Input: part model. Units: mm. Frame: model coordinates. A direction names the side the tool comes from. Coordinates: 2 decimals unless noted, no trailing zeros. Order: outer loops, then holes, each group sorted by start corner. A loop starts at its lowest first (then second) coordinate and runs counter-clockwise, first axis right, second up. Notation, with made-up numbers: (55, 51) -> (67, 51) arc R19 ccw to (67, 57) -> close; hole circle Ø4 at (-24.5, 43.25). An arc over 180 degrees is marked (long way). Use CSV: the item, a comma, the result in double quotes. Start each with the question number.
```python
from build123d import *

# Parameters (mm, degrees)
F0_R     = 25.4
F0_R_2   = 1.5875
F1_DEPTH = 3.175


with BuildPart() as f1:
    # F0 (on Top) → F1 (new body)
    with BuildSketch(Plane.XY):
        Circle(F0_R)
        with BuildLine():
            ThreePointArc((15.7154482119, 15.7154482119), (20.5332226101, 8.5051392843), (22.225, 0))
            ThreePointArc((22.225, 0), (20.5332226101, -8.5051392843), (15.7154482119, -15.7154482119))
            ThreePointArc((15.7154482119, -15.7154482119), (8.5051392843, -20.5332226101), (0, -22.225))
            ThreePointArc((0, -22.225), (-8.5051392843, -20.5332226101), (-15.7154482119, -15.7154482119))
            ThreePointArc((-15.7154482119, -15.7154482119), (-20.5332226101, -8.5051392843), (-22.225, 0))
            ThreePointArc((-22.225, 0), (-20.5332226101, 8.5051392843), (-15.7154482119, 15.7154482119))
            ThreePointArc((-15.7154482119, 15.7154482119), (-8.5051392843, 20.5332226101), (0, 22.225))
            ThreePointArc((0, 22.225), (8.5051392843, 20.5332226101), (15.7154482119, 15.7154482119))
        make_face(mode=Mode.SUBTRACT)
        with BuildLine():
            Line((0, 6.35), (0, 22.225))
            ThreePointArc((0, 22.225), (-8.5051392843, 20.5332226101), (-15.7154482119, 15.7154482119))
            Line((-15.7154482119, 15.7154482119), (-4.4901280605, 4.4901280605))
            ThreePointArc((-4.4901280605, 4.4901280605), (-2.4300397955, 5.8666350314), (0, 6.35))
        make_face()
        with BuildLine():
            Line((6.35, 0), (22.225, 0))
            ThreePointArc((22.225, 0), (20.5332226101, 8.5051392843), (15.7154482119, 15.7154482119))
            Line((15.7154482119, 15.7154482119), (4.4901280605, 4.4901280605))
            ThreePointArc((4.4901280605, 4.4901280605), (5.8666350314, 2.4300397955), (6.35, 0))
        make_face()
        with BuildLine():
            ThreePointArc((0, -22.225), (8.5051392843, -20.5332226101), (15.7154482119, -15.7154482119))
            Line((15.7154482119, -15.7154482119), (4.4901280605, -4.4901280605))
            ThreePointArc((4.4901280605, -4.4901280605), (2.4300397955, -5.8666350314), (0, -6.35))
            Line((0, -6.35), (0, -22.225))
        make_face()
        with BuildLine():
            ThreePointArc((-22.225, 0), (-20.5332226101, -8.5051392843), (-15.7154482119, -15.7154482119))
            Line((-15.7154482119, -15.7154482119), (-4.4901280605, -4.4901280605))
            ThreePointArc((-4.4901280605, -4.4901280605), (-5.8666350314, -2.4300397955), (-6.35, 0))
            Line((-6.35, 0), (-22.225, 0))
        make_face()
        with BuildLine():
            ThreePointArc((4.4901280605, -4.4901280605), (5.8666350314, -2.4300397955), (6.35, 0))
            ThreePointArc((6.35, 0), (5.8666350314, 2.4300397955), (4.4901280605, 4.4901280605))
            ThreePointArc((4.4901280605, 4.4901280605), (2.4300397955, 5.8666350314), (0, 6.35))
            ThreePointArc((0, 6.35), (-2.4300397955, 5.8666350314), (-4.4901280605, 4.4901280605))
            ThreePointArc((-4.4901280605, 4.4901280605), (-5.8666350314, 2.4300397955), (-6.35, 0))
            ThreePointArc((-6.35, 0), (-5.8666350314, -2.4300397955), (-4.4901280605, -4.4901280605))
            ThreePointArc((-4.4901280605, -4.4901280605), (-2.4300397955, -5.8666350314), (0, -6.35))
            ThreePointArc((0, -6.35), (2.4300397955, -5.8666350314), (4.4901280605, -4.4901280605))
        make_face()
        Circle(F0_R_2, mode=Mode.SUBTRACT)
    extrude(amount=F1_DEPTH)


solid = f1.part
```
1. Pull-direction query (Y, two-part tool) for faces 1 (the face through (20.58, -8.39, 1.57)), 2 (the face through (-5.506, -24.796, 1.565)), 3 (the face through (5, 0, 0)), 4 (the face through (-2.462, -5.853, 1.565)); classes: released by +Y, released by -Y, zero draft, split by the parting line, or undercut.
2. Section B-B on x = -1. Return loops of the section in (y, z) (1 decimal), then the cut area to 3 significant figures.
3. Access query for faces 5 (the face through (-20.58, 8.39, 1.57)), 6 (the face through (5, 0, 3.175)). Directions: +Z, -Z, +X, -X, +Y, -Y. A direction counts if a zero-diameter tool reaches every point of the face in a straight line with its end or side. Return the directions, or none.
4. Section C-C on y = -19. Return loops of the section in (x, z) (3 decimals).
5. Contact query for flat-ended pins moving along their axis: P1, Ø2.5, axis at x = 0, y = 0, coming from the +Z side; P2, Ø1, axis at x = -6, z = 2.5, coming from the +Y side; P3, Ø1, axis at y = -14.5, z = 2, coming from the -X side; P4, Ø1.6, axis at x = -12.5, z = 1, coming from the +Y side. Output: stop coordinate, or through.
6. Material intervals for line 1 along X through (y, z) = (-10, 0.3); line 2 along X through (y, z) = (-11, 2.65); line 3 along Y through (x, z) = (-6.5, 0.85), sorted ascending.
7. Section D-D on y = -9. Return loops of the section in (x, z) (3 decimals), then the cut area to 3 significant figures.
8. Section A-A on z = 1.7. State how many separate pieces and enclosed holes the cut face has, then the cut area to 3 significant figures.
Values follow:
1,face 1,"undercut"
1,face 2,"split by the parting line"
1,face 3,"zero draft"
1,face 4,"undercut"
2,outline,"(-25.4, 0) -> (-22.2, 0) -> (-22.2, 3.2) -> (-25.4, 3.2) -> close; (-6.3, 0) -> (-1.2, 0) -> (-1.2, 3.2) -> (-6.3, 3.2) -> close; (1.2, 0) -> (25.4, 0) -> (25.4, 3.2) -> (1.2, 3.2) -> close"
2,area,"103 mm2"
3,face 5,"+Z, -Z"
3,face 6,"+Z, +X, -X, +Y, -Y"
4,outline,"(-16.857, 0) -> (-11.53, 0) -> (-11.53, 3.175) -> (-16.857, 3.175) -> close; (0, 0) -> (16.857, 0) -> (16.857, 3.175) -> (0, 3.175) -> close"
5,P1,"passes through"
5,P2,"stops at y = 24.8"
5,P3,"stops at x = -21.19"
5,P4,"stops at y = 22.54"
6,line 1,"x = -23.35 to -10, 0 to 10, 19.85 to 23.35"
6,line 2,"x = -22.89 to -11, 0 to 11, 19.31 to 22.89"
6,line 3,"y = -24.55 to -21.25, -6.5 to 0, 6.5 to 24.55"
7,outline,"(-23.752, 0) -> (-9, 0) -> (-9, 3.175) -> (-23.752, 3.175) -> close; (0, 0) -> (9, 0) -> (9, 3.175) -> (0, 3.175) -> close; (20.321, 0) -> (23.752, 0) -> (23.752, 3.175) -> (20.321, 3.175) -> close"
7,area,"86.3 mm2"
8,separate pieces,"1"
8,enclosed holes,"5"
8,area,"1,310 mm2"
